Could you check a few things on this model? Use its own coordinates, in mm. A direction names the side the tool comes from. Coordinates: 2 decimals unless noted, no trailing zeros. Loops run counter-clockwise (first coordinate to the right, second up) from the corner with the lowest first, then second, coordinate; pieces in that order, holes last.
from build123d import *

# Parameters (mm, degrees)
SALIENTE_EXTRUIR1_DEPTH = 3
CORTAR_EXTRUIR1_REACH   = 36.517
CROQUIS2_R              = 1.5
CROQUIS2_R_2            = 1.002612495
CORTAR_EXTRUIR2_START   = -3
CROQUIS3_W              = 3
CROQUIS3_H              = 35
CORTAR_EXTRUIR2_DEPTH   = 3
CROQUIS4_W              = 3
CROQUIS4_H              = 8
SALIENTE_EXTRUIR2_DEPTH = 3


with BuildPart() as part:
    # Croquis1 → Saliente-Extruir1 (new body)
    with BuildSketch(Plane.XY):
        Polygon((29.6, -12.5), (26.6, -12.5), (26.6, -7.5), (29.6, -7.5), (29.6, -2.5), (26.6, -2.5), (26.6, 2.5), (29.6, 2.5), (29.6, 7.5), (26.6, 7.5), (26.6, 12.5), (29.6, 12.5), (29.6, 17.5), (-29.6, 17.5), (-29.6, 12.5), (-26.6, 12.5), (-26.6, 7.5), (-29.6, 7.5), (-29.6, 2.5), (-26.6, 2.5), (-26.6, -2.5), (-29.6, -2.5), (-29.6, -7.5), (-26.6, -7.5), (-26.6, -12.5), (-29.6, -12.5), (-29.6, -17.5), (29.6, -17.5), align=None)
    extrude(amount=SALIENTE_EXTRUIR1_DEPTH)

    # Croquis2 → Cortar-Extruir1 (cut, up to next)
    with BuildSketch(Plane(origin=(0, 0, 0), x_dir=(-1, 0, 0), z_dir=(0, 0, -1)), mode=Mode.PRIVATE) as cortar_extruir1_sk1:
        with Locations((-7.6, 0.31)):
            Circle(CROQUIS2_R)
    cortar_extruir1_tool1 = extrude(cortar_extruir1_sk1.sketch, amount=-CORTAR_EXTRUIR1_REACH, mode=Mode.PRIVATE) & part.part
    # Croquis2 → Cortar-Extruir1 (cut, up to next)
    with BuildSketch(Plane(origin=(0, 0, 0), x_dir=(-1, 0, 0), z_dir=(0, 0, -1)), mode=Mode.PRIVATE) as cortar_extruir1_sk2:
        with Locations((-15.1, 0.31)):
            Circle(CROQUIS2_R_2)
    cortar_extruir1_tool2 = extrude(cortar_extruir1_sk2.sketch, amount=-CORTAR_EXTRUIR1_REACH, mode=Mode.PRIVATE) & part.part
    # Croquis2 → Cortar-Extruir1 (cut, up to next)
    with BuildSketch(Plane(origin=(0, 0, 0), x_dir=(-1, 0, 0), z_dir=(0, 0, -1)), mode=Mode.PRIVATE) as cortar_extruir1_sk3:
        with Locations((-11.35, 6.805190528)):
            Circle(CROQUIS2_R_2)
    cortar_extruir1_tool3 = extrude(cortar_extruir1_sk3.sketch, amount=-CORTAR_EXTRUIR1_REACH, mode=Mode.PRIVATE) & part.part
    # Croquis2 → Cortar-Extruir1 (cut, up to next)
    with BuildSketch(Plane(origin=(0, 0, 0), x_dir=(-1, 0, 0), z_dir=(0, 0, -1)), mode=Mode.PRIVATE) as cortar_extruir1_sk4:
        with Locations((-3.85, 6.805190528)):
            Circle(CROQUIS2_R_2)
    cortar_extruir1_tool4 = extrude(cortar_extruir1_sk4.sketch, amount=-CORTAR_EXTRUIR1_REACH, mode=Mode.PRIVATE) & part.part
    # Croquis2 → Cortar-Extruir1 (cut, up to next)
    with BuildSketch(Plane(origin=(0, 0, 0), x_dir=(-1, 0, 0), z_dir=(0, 0, -1)), mode=Mode.PRIVATE) as cortar_extruir1_sk5:
        with Locations((-0.1, 0.31)):
            Circle(CROQUIS2_R_2)
    cortar_extruir1_tool5 = extrude(cortar_extruir1_sk5.sketch, amount=-CORTAR_EXTRUIR1_REACH, mode=Mode.PRIVATE) & part.part
    # Croquis2 → Cortar-Extruir1 (cut, up to next)
    with BuildSketch(Plane(origin=(0, 0, 0), x_dir=(-1, 0, 0), z_dir=(0, 0, -1)), mode=Mode.PRIVATE) as cortar_extruir1_sk6:
        with Locations((-3.85, -6.185190528)):
            Circle(CROQUIS2_R_2)
    cortar_extruir1_tool6 = extrude(cortar_extruir1_sk6.sketch, amount=-CORTAR_EXTRUIR1_REACH, mode=Mode.PRIVATE) & part.part
    # Croquis2 → Cortar-Extruir1 (cut, up to next)
    with BuildSketch(Plane(origin=(0, 0, 0), x_dir=(-1, 0, 0), z_dir=(0, 0, -1)), mode=Mode.PRIVATE) as cortar_extruir1_sk7:
        with Locations((-11.35, -6.185190528)):
            Circle(CROQUIS2_R_2)
    cortar_extruir1_tool7 = extrude(cortar_extruir1_sk7.sketch, amount=-CORTAR_EXTRUIR1_REACH, mode=Mode.PRIVATE) & part.part
    add(cortar_extruir1_tool1.solids().sort_by_distance((7.6, 0.31, 0))[0], mode=Mode.SUBTRACT)
    add(cortar_extruir1_tool2.solids().sort_by_distance((15.1, 0.31, 0))[0], mode=Mode.SUBTRACT)
    add(cortar_extruir1_tool3.solids().sort_by_distance((11.35, 6.805191, 0))[0], mode=Mode.SUBTRACT)
    add(cortar_extruir1_tool4.solids().sort_by_distance((3.85, 6.805191, 0))[0], mode=Mode.SUBTRACT)
    add(cortar_extruir1_tool5.solids().sort_by_distance((0.1, 0.31, 0))[0], mode=Mode.SUBTRACT)
    add(cortar_extruir1_tool6.solids().sort_by_distance((3.85, -6.185191, 0))[0], mode=Mode.SUBTRACT)
    add(cortar_extruir1_tool7.solids().sort_by_distance((11.35, -6.185191, 0))[0], mode=Mode.SUBTRACT)

    # Croquis3 → Cortar-Extruir2 (cut)
    with BuildSketch(Plane.XY.offset(3).offset(CORTAR_EXTRUIR2_START)):
        with Locations((-28.1, 0)):
            Rectangle(CROQUIS3_W, CROQUIS3_H)
        with Locations((28.1, 0)):
            Rectangle(CROQUIS3_W, CROQUIS3_H)
    extrude(amount=CORTAR_EXTRUIR2_DEPTH, mode=Mode.SUBTRACT)

    # Croquis4 → Saliente-Extruir2 (add)
    with BuildSketch(Plane.XY.offset(3)):
        with Locations((28.1, 0)):
            Rectangle(CROQUIS4_W, CROQUIS4_H)
        with Locations((-28.1, 0)):
            Rectangle(CROQUIS4_W, CROQUIS4_H)
    extrude(amount=-SALIENTE_EXTRUIR2_DEPTH)


solid = part.part
(1) Which directions (+Z, -Z, +X, -X, +Y, -Y) give clear straight access to the entire face, cutting with the end or side of a thin tool? Please do faces 1 (the face through (26.6, 11, 1)), 2 (the face through (3.98, 7.8, 1.48)), 3 (the face through (-28, 4, 2)), 4 (the face through (-26.6, -11, 1)).
Answers:
face 1: +Z, -Z, +X, +Y
face 2: +Z, -Z
face 3: +Z, -Z, -X, +Y
face 4: +Z, -Z, -X, -Y
(2) Imagine slicing it at A-A, the plane x = 3.85. Write out the boundary of the cut face in (y, z), and give its area (3 significant figures).
Answers:
outline: (-17.5, 0) - (-7.19, 0) - (-7.19, 3) - (-17.5, 3) - close; (-5.18, 0) - (5.8, 0) - (5.8, 3) - (-5.18, 3) - close; (7.81, 0) - (17.5, 0) - (17.5, 3) - (7.81, 3) - close
area: 93.0 mm2
(3) We'd pull the mould along Y, two halves only. Please class faces 5 (the face through (26.6, -11, 1)), 6 (the face through (-0.856, 0.611, 1.479)), 7 (the face through (28, -4, 2)): +Y half, -Y half, draft (parallel to the pull), parting line (faces both ways), or undercut.
Answers:
face 5: draft
face 6: undercut
face 7: -Y half
(4) Imagine slicing it at B-B, the plane y = 0.31. Write out the boundary of the cut face in (x, z).
Answers:
outline: (-29.6, 0) - (-0.9, 0) - (-0.9, 3) - (-29.6, 3) - close; (1.1, 0) - (6.1, 0) - (6.1, 3) - (1.1, 3) - close; (9.1, 0) - (14.1, 0) - (14.1, 3) - (9.1, 3) - close; (16.1, 0) - (29.6, 0) - (29.6, 3) - (16.1, 3) - close
(5) Imagine slicing it at C-C, the plane z = 1.8. Write out the boundary of the cut face in (x, y).
Answers:
outline: (-29.6, -4) - (-26.6, -4) - (-26.6, -17.5) - (26.6, -17.5) - (26.6, -4) - (29.6, -4) - (29.6, 4) - (26.6, 4) - (26.6, 17.5) - (-26.6, 17.5) - (-26.6, 4) - (-29.6, 4) - close; hole circle Ø2.01 at (0.1, 0.31); hole circle Ø2.01 at (3.85, -6.19); hole circle Ø2.01 at (3.85, 6.81); hole circle Ø3 at (7.6, 0.31); hole circle Ø2.01 at (11.35, -6.19); hole circle Ø2.01 at (11.35, 6.81); hole circle Ø2.01 at (15.1, 0.31)
(6) I need wall thicknesses on probe 1 along Y at (x, z) = (11.35, 1.9); probe 2 along X at (y, z) = (-6, 1.95); probe 3 along X at (y, z) = (7.5, 0.15). Which ranges of each line are inside material? Lowest first, please.
Answers:
probe 1: y = -17.5 to -7.19, -5.18 to 5.8, 7.81 to 17.5
probe 2: x = -26.6 to 2.86, 4.84 to 10.36, 12.34 to 26.6
probe 3: x = -26.6 to 3.13, 4.57 to 10.63, 12.07 to 26.6
(7) For pin 1 (0.9 mm diameter, centred on x = 27.5, z = 2, fed in from -Y); pin 2 (1.5 mm diameter, centred on y = 11.5, z = 1, fed in from +X); pin 3 (0.9 mm diameter, centred on y = 14, z = 1.5, fed in from -X), each with a flat end and sliding along its axis, tell me the tip position at first contact or that it passes through.
Answers:
pin 1: stops at y = -4
pin 2: stops at x = 26.6
pin 3: stops at x = -26.6
